Geometry: see drawing. Coordinates: mm, zero at the bounding-box minimum. A direction names the side the tool comes from. Coordinates: 2 decimals unless noted, no trailing zeros. Write each loop counter-clockwise with the first axis right and the second up, starting at its lowest first coordinate (ties: lowest second). Pieces come first, ordered by that corner, then holes. Notation, with made-up numbers: (-33, -27) - (-25, -27) arc R27 cw to (-25, 12) - close; hole circle Ø11 at (69.5, 67.25). An arc over 180 degrees is marked (long way). One line per question, with ' | ' between items. Start each with the question number.
1) Section query B-B on y = 23. Return loops of the section in (x, z) (3 decimals), and give its area (3 significant figures).
2) Section query C-C on z = 54. Return loops of the section in (x, y), and give its area (3 significant figures).
3) Line query: line 1 (Z direction, x = 217.5, y = 73.5) (3 decimals); line 2 (Z direction, x = 379.5, y = 36.5) (3 decimals); line 3 (X direction, y = 82, z = 53). Output: solid intervals per line, ascending.
4) Section query A-A on x = 403. Return loops of the section in (y, z) (3 decimals).
5) First-contact query: P1, Ø1, axis at y = 15, z = 70.5, coming from the -X side; P2, Ø1, axis at y = 46.5, z = 34.5, coming from the +X side (3 decimals); P3, Ø5, axis at x = 352, y = 63, coming from the -Z side. Flat tips, straight axial feed; report the tip coordinate or a pass-through.
6) Reachability of the marked faces 1, 2 and 3 from +Z, -Z, +X, -X, +Y, -Y: full face, straight path, thin tool, end or side. Return the list, or none.
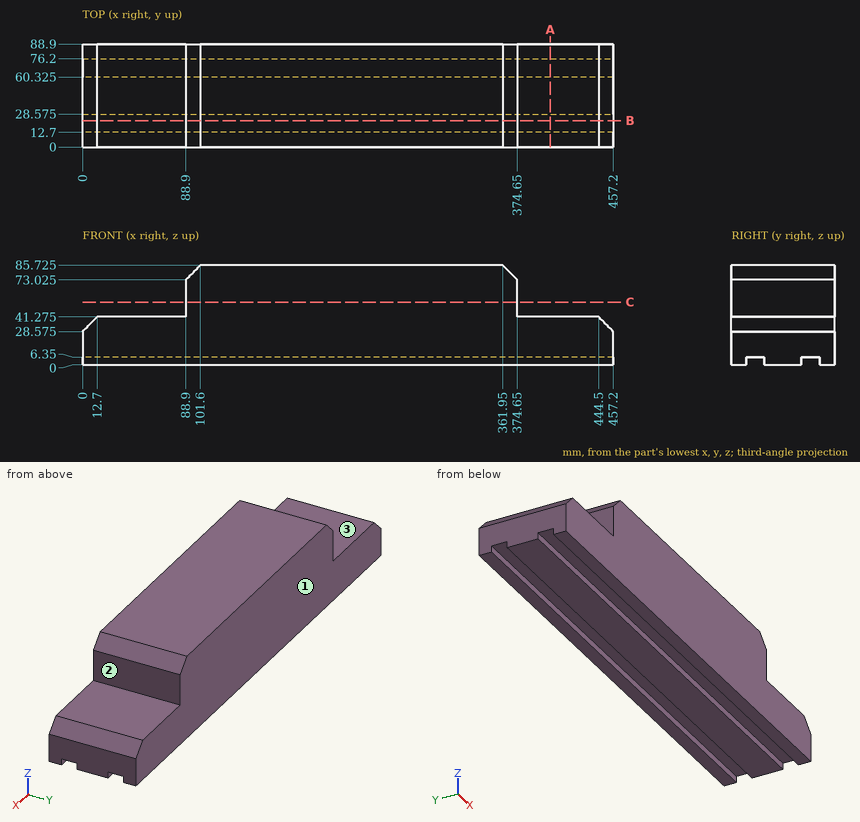
Answer key:
1) outline: (0, 6.35) - (457.2, 6.35) - (457.2, 28.575) - (444.5, 41.275) - (374.65, 41.275) - (374.65, 73.025) - (361.95, 85.725) - (101.6, 85.725) - (88.9, 73.025) - (88.9, 41.275) - (12.7, 41.275) - (0, 28.575) - close | area: 28,300 mm²
2) outline: (88.9, 0) - (374.65, 0) - (374.65, 88.9) - (88.9, 88.9) - close | area: 25,400 mm²
3) line 1: 6.35 to 85.725 | line 2: 0 to 41.275 | line 3: 88.9 to 374.65
4) outline: (0, 0) - (12.7, 0) - (12.7, 6.35) - (28.575, 6.35) - (28.575, 0) - (60.325, 0) - (60.325, 6.35) - (76.2, 6.35) - (76.2, 0) - (88.9, 0) - (88.9, 41.275) - (0, 41.275) - close
5) P1: x = 88.9 | P2: x = 451.775 | P3: z = 6.35
6) face 1: +Z, -Z, +X, -X, +Y | face 2: +Z, +X, +Y, -Y | face 3: +Z, -X, +Y, -Y
